The figure shows three views and two pictorial views of one solid part (mm, origin at its lowest corner). Answer the questions. A direction names the side the tool comes from. Coordinates: 2 decimals unless noted, no trailing zeros. Order: outer loops, then holes, each group sorted by start corner. A loop starts at its lowest first (then second) coordinate and runs counter-clockwise, first axis right, second up. Notation, with made-up numbers: (51, -9.75) -> (107, -9.75) arc R16 cw to (107, 15.25) -> close; hole circle Ø3 at (6.5, -21). An arc over 180 degrees is marked (long way). Return JSON: item names as keys, results as strings.
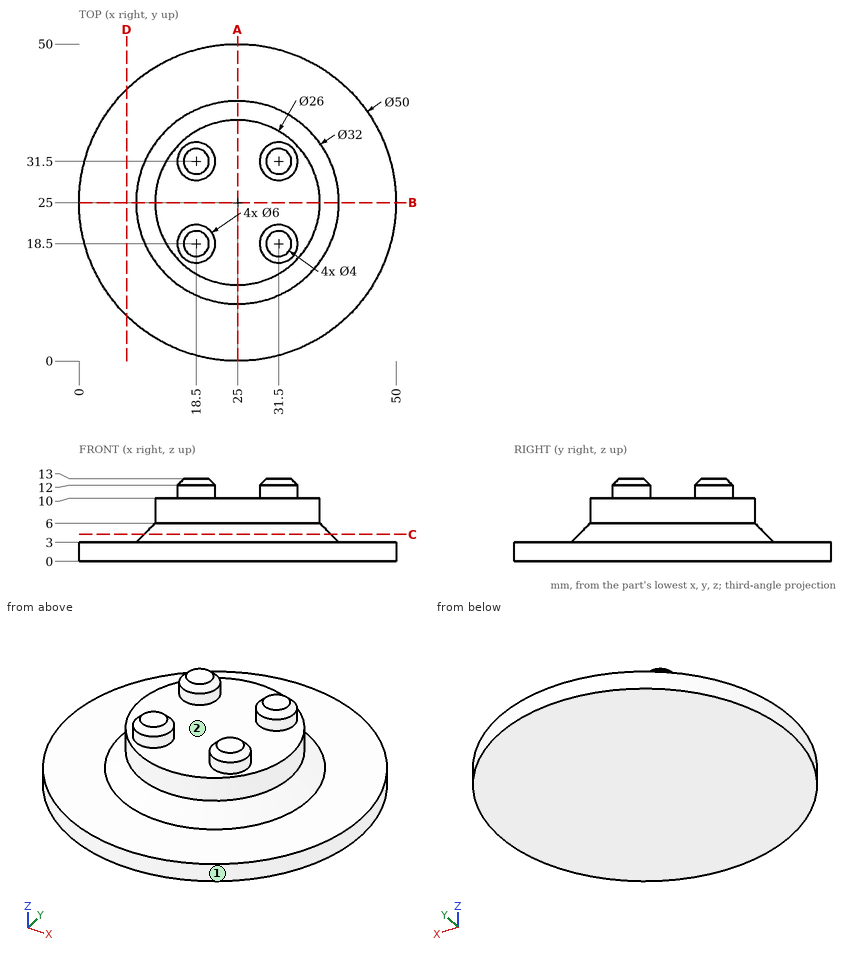
Item 1: Find the intervals of material crossed by probe 1 along Z at (x, y) = (14, 4); probe 2 along Y at (x, z) = (19, 11.5); probe 3 along X at (y, z) = (29.5, 12), in increasing order.
Answer list:
{"probe 1": "0 to 3", "probe 2": "15.54 to 21.46, 28.54 to 34.46", "probe 3": "16.26 to 20.74, 29.26 to 33.74"}
Item 2: The part is cut by section C-C on z = 4.25. Determine the outline of the cut face in (x, y), plus the area to 3 significant figures.
Answer list:
{"outline": "circle Ø29.5 at (25, 25)", "area": "683 mm2"}
Item 3: Flat-ended cylindrical pins translate along their axes: pin 1 (6 mm diameter, centred on y = 42, z = 5.5, fed in from +X); pin 2 (12 mm diameter, centred on x = 39, y = 43, fed in from -Z); pin 3 (4 mm diameter, centred on x = 15.5, z = 11.5, fed in from +Y); pin 4 (8 mm diameter, centred on x = 5.5, y = 42.5, fed in from +Z). Find the tip coordinate at first contact, or state that the pin passes through.
Answer list:
{"pin 1": "x = 44.74", "pin 2": "z = 0", "pin 3": "y = 35.11", "pin 4": "z = 3"}
Item 4: The part is cut by section D-D on x = 7.5. Determine the outline of the cut face in (y, z).
Answer list:
{"outline": "(7.15, 0) -> (42.85, 0) -> (42.85, 3) -> (7.15, 3) -> close"}
Item 5: Which of the six approach directions +Z, -Z, +X, -X, +Y, -Y give full straight-line access (tool end or side, diameter ignored) to the marked faces 1 and 2?
Answer list:
{"face 1": "+Z, -Z", "face 2": "+Z"}
Item 6: The part is cut by section A-A on x = 25. Determine the outline of the cut face in (y, z), plus the area to 3 significant figures.
Answer list:
{"outline": "(0, 0) -> (50, 0) -> (50, 3) -> (41, 3) -> (38, 6) -> (38, 10) -> (12, 10) -> (12, 6) -> (9, 3) -> (0, 3) -> close", "area": "341 mm2"}
